```python
from build123d import *

# Parameters (mm, degrees)
F2_W     = 0.508
F2_H     = 0.942
F2_W_2   = 0.942
F2_H_2   = 0.508
F3_DEPTH = 0.254
F3_TAPER = -3
F4_SIZE  = 0.508


with BuildPart() as f1:
    # F0 (on Front) → F1 (revolve)
    with BuildSketch(Plane.XZ):
        Polygon((0, 13), (0, 0), (1.25, 0), (1.25, 11.9), (2.35, 13), align=None)
    revolve(axis=Axis((0, 0, 6.5), (0, 0, 1)))

    # F2 (on face) → F3 (cut)
    with BuildSketch(Plane.XY.offset(13)):
        Polygon((-0.508, 0.1779751724), (-1.45, 0.508), (-1.45, 0), (-0.508, 0), align=None)
        Polygon((-0.508, 0.508), (-1.45, 0.508), (-0.508, 0.1779751724), align=None)
        with Locations((-0.254, 0.979)):
            Rectangle(F2_W, F2_H)
        Polygon((0, 0.508), (-0.508, 0.508), (-0.508, 0.1779751724), (0, 0), align=None)
        with Locations((-0.979, -0.254)):
            Rectangle(F2_W_2, F2_H_2)
        Polygon((0, 1.45), (0, 0.508), (0.1779751724, 0.508), (0.508, 1.45), align=None)
        Polygon((0, 0), (-0.508, 0), (-0.508, -0.508), (-0.1779751724, -0.508), align=None)
        Polygon((0.508, -0.1779751724), (0, 0), (0, -0.508), (0.508, -0.508), align=None)
        Polygon((0.1779751724, 0.508), (0, 0), (0.508, 0), (0.508, 0.508), align=None)
        Polygon((0.508, 1.45), (0.1779751724, 0.508), (0.508, 0.508), align=None)
        Polygon((-0.1779751724, -0.508), (-0.508, -0.508), (-0.508, -1.45), align=None)
        Polygon((0, -1.45), (0, -0.508), (-0.1779751724, -0.508), (-0.508, -1.45), align=None)
        with Locations((0.254, -0.979)):
            Rectangle(F2_W, F2_H)
        Polygon((1.45, 0), (0.508, 0), (0.508, -0.1779751724), (1.45, -0.508), align=None)
        with Locations((0.979, 0.254)):
            Rectangle(F2_W_2, F2_H_2)
        Polygon((1.45, -0.508), (0.508, -0.1779751724), (0.508, -0.508), align=None)
        Polygon((0.1779751724, 0.508), (0, 0.508), (0, 0), align=None)
        Polygon((0.508, 0), (0, 0), (0.508, -0.1779751724), align=None)
        Polygon((0, -0.508), (0, 0), (-0.1779751724, -0.508), align=None)
        Polygon((0, 0), (-0.508, 0.1779751724), (-0.508, 0), align=None)
    extrude(amount=-F3_DEPTH, taper=F3_TAPER, mode=Mode.SUBTRACT)

    # F4
    f4_edges = [f1.edges().sort_by_distance(p)[0] for p in [
        (-1.25, 0, 0),
    ]]
    chamfer(f4_edges, length=F4_SIZE)


solid = f1.part
```
Input: part model. Units: mm. Frame: model coordinates. Give positions to 0.01 mm unless a question says otherwise; leave off trailing zeros. Loops run counter-clockwise (first coordinate to the right, second up) from the corner with the lowest first, then second, coordinate; pieces in that order, holes last.
1) Contact query for flat-ended pins moving along their axis: pin 1 (1.5 mm diameter, centred on x = 0, z = 10.5, fed in from +Y); pin 2 (1.5 mm diameter, centred on y = 1.5, z = 1.5, fed in from -X); pin 3 (1.5 mm diameter, centred on y = -0.5, z = 8, fed in from -X). Output: stop coordinate, or through.
A:
pin 1: stops at y = 1.25
pin 2: stops at x = -1
pin 3: stops at x = -1.25
2) Section query A-A on z = 5.25. Return the cut outline in (x, y), and give its area (3 significant figures).
A:
outline: circle Ø2.5 at (0, 0)
area: 4.91 mm2
3) Line query: L1, parallel to Z at x = -0.45, y = -0.5; L2, parallel to Y at x = 0, z = 3.25; L3, parallel to Y at x = 0.85, z = 6.75. Output: solid intervals per line, ascending.
A:
L1: z = 0 to 12.75
L2: y = -1.25 to 1.25
L3: y = -0.92 to 0.92
4) Mould query, pull axis X, two halves, no side actions, for faces 1 (the flat face through (0, 0, 12.746)), 2 (the cylindrical face through (-0.27, -1.22, 6.28)), 3 (the flat face through (-1, 1, 13)). Classes: released by +X, released by -X, zero draft, split by the parting line, or undercut.
A:
face 1: undercut
face 2: split by the parting line
face 3: zero draft
